Verification items for the finished model (mm, model axes). A direction names the side the tool comes from. Round coordinates to 2 decimals unless told otherwise and drop trailing zeros. Write each loop counter-clockwise with the first axis right and the second up, starting at its lowest first coordinate (ties: lowest second). Pieces come first, ordered by that corner, then holes. Notation, with made-up numbers: M 6,0.25 L 25,0.25 A34 cw 25,31.25 Z; hole C 16,-15.75 d6. An arc over 180 degrees is marked long. One line per question, with ' | ' between items.
from build123d import *

# Parameters (mm, degrees)
PAD_DEPTH    = 6
SKETCH001_R  = 10
PAD001_DEPTH = 50
PAD001_TAPER = 7.180756
FILLET_R     = 2
FILLET001_R  = 1


with BuildPart() as part:
    # Sketch → Pad (new body)
    with BuildSketch(Plane.XY):
        with BuildLine():
            Line((15, -25), (-15, -25))
            ThreePointArc((-25, -15), (-22.071068, -22.071068), (-15, -25))
            Line((-25, -15), (-25, 15))
            ThreePointArc((-15, 25), (-22.071068, 22.071068), (-25, 15))
            Line((-15, 25), (15, 25))
            ThreePointArc((25, 15), (22.071068, 22.071068), (15, 25))
            Line((25, 15), (25, -15))
            ThreePointArc((15, -25), (22.071068, -22.071068), (25, -15))
        make_face()
    extrude(amount=PAD_DEPTH)

    # Sketch001 (on Face10 of Pad) → Pad001 (join)
    with BuildSketch(Plane.XY.offset(6)):
        Circle(SKETCH001_R)
    extrude(amount=PAD001_DEPTH, taper=PAD001_TAPER)

    # Fillet
    fillet_edges = [part.edges().sort_by_distance(p)[0] for p in [
        (-10, 0, 6),
    ]]
    fillet(fillet_edges, radius=FILLET_R)

    # Fillet001
    fillet001_edges = [part.edges().sort_by_distance(p)[0] for p in [
        (-3.700592, 0, 56),
    ]]
    fillet(fillet001_edges, radius=FILLET001_R)


solid = part.part
1. Go/stop test with flat-tipped pins: P1, Ø10, axis at y = -14, z = 45.5, coming from the +X side; P2, Ø8, axis at x = 17.5, y = -0.5, coming from the +Z side. Record where each tip stops, or that it passes through.
Results:
P1: passes through | P2: stops at z = 6
2. Thickness scan on line 1 (Z direction, x = 22.5, y = 8.5); line 2 (Y direction, x = -1, z = 50); line 3 (Y direction, x = 4, z = 28.5). Record the ranges inside material, lowest first.
Results:
line 1: z = 0 to 6 | line 2: y = -4.34 to 4.34 | line 3: y = -5.94 to 5.94
3. Section check A-A, the plane x = 0. Record the cut outline in (y, z) (3 decimals), then the cut area to 3 significant figures.
Results:
outline: M -25,0 L 25,0 L 25,6 L 11.764,6 A2 cw 9.78,7.75 L 3.811,55.125 A1 ccw 2.819,56 L -2.819,56 A1 ccw -3.811,55.125 L -9.78,7.75 A2 cw -11.764,6 L -25,6 Z | area: 986 mm2
4. Section check D-D, the plane y = 13.5. Record the cut outline in (x, z).
Results:
outline: M -25,0 L 25,0 L 25,6 L -25,6 Z
5. Tool access check on faces 1 (the face through (-11, -5, 6)), 2 (the face through (22.15, 21.99, 2.96)). Record the directions out of +Z, -Z, +X, -X, +Y, -Y that give a thin tool (end or side, any length) a straight path to the whole face; none if there is none.
Results:
face 1: +Z | face 2: +Z, -Z, +X, +Y
6. Section check C-C, the plane z = 24. Record the cut outline in (x, y), then the cut area to 3 significant figures.
Results:
outline: C 0,0 d15.46 | area: 188 mm2
